Geometry: final body of the model. Coordinates: model frame, mm. A direction names the side the tool comes from. Give positions to 0.01 mm unless a question says otherwise; leave off trailing zeros. Write each loop counter-clockwise with the first axis right and the second up, starting at its lowest first coordinate (ties: lowest second). Pieces come first, ordered by that corner, then holes.
Q1. Cut plane A-A on z = 0. Return the cut outline in (x, y), plus the area to 3 significant figures.
Q2. Reachability of faces 1 (the face through (-7.5, 6, 2)), 2 (the face through (-2.81, 1, 0)), 3 (the face through (-6, 4, 10)) from +Z, -Z, +X, -X, +Y, -Y: full face, straight path, thin tool, end or side. Return the list, or none.
Q3. Cut plane D-D on x = 1.5. Return the cut outline in (y, z), plus the area to 3 significant figures.
Q4. Cut plane B-B on x = -8. Return the cut outline in (y, z), plus the area to 3 significant figures.
Q5. Line query: L1, parallel to Z at x = -9, y = 6; L2, parallel to Y at x = -8.15, z = 0; L3, parallel to Z at x = -6.75, y = 8.25. Output: solid intervals per line, ascending.
Q6. Cut plane C-C on y = 6. Return the cut outline in (x, z).
Q7. Pin query (flat end, axial travel): pin 1 (3.5 mm diameter, centred on y = 6, z = -4, fed in from +X); pin 2 (9 mm diameter, centred on x = 2, z = -2, fed in from +Y). Return the tip coordinate at first contact, or that it passes through.
Q8. Draft query along Y for faces 4 (the face through (-9, 10, 0)), 5 (the face through (-5, 4, -8)), 6 (the face through (-8.73, 6.97, -5.27)). Return one class per face: pulls with the +Y half, pulls with the -Y half, needs draft (parallel to the pull), parting line crosses it, or undercut.
```python
from build123d import *

# Parameters (mm, degrees)
SKETCH1_R           = 3.1
BOSS_EXTRUDE1_DEPTH = 2
BOSS_EXTRUDE2_DEPTH = 10
BOSS_EXTRUDE3_DEPTH = 2
BOSS_EXTRUDE4_DEPTH = 2
CUT_EXTRUDE1_DEPTH  = 5
BOSS_EXTRUDE5_START = -2
BOSS_EXTRUDE5_DEPTH = 2


with BuildPart() as part:
    # Sketch1 → Boss-Extrude1 (new body)
    with BuildSketch(Plane(origin=(0, 0, 0), x_dir=(1, 0, 0), z_dir=(0, 1, 0))):
        with BuildLine():
            ThreePointArc((0, -10), (10, 0), (0, 10))
            Line((0, 10), (-10, 10))
            Line((-10, 10), (-10, -10))
            Line((-10, -10), (0, -10))
        make_face()
        with Locations(Location((0, 0, 0), (0, 0, 270))):
            Circle(SKETCH1_R, mode=Mode.SUBTRACT)
    extrude(amount=BOSS_EXTRUDE1_DEPTH)

    # Sketch1<3> → Boss-Extrude2 (add)
    with BuildSketch(Plane(origin=(0, 0, 0), x_dir=(1, 0, 0), z_dir=(0, 1, 0))):
        with BuildLine():
            Line((-7.5, -6.614378278), (-7.5, 6.614378278))
            ThreePointArc((-7.5, 6.614378278), (-9.354143467, 3.535533906), (-10, 0))
            ThreePointArc((-10, 0), (-9.354143467, -3.535533906), (-7.5, -6.614378278))
        make_face()
        with BuildLine():
            Line((-7.5, 6.614378278), (-7.5, 10))
            Line((-7.5, 10), (-10, 10))
            Line((-10, 10), (-10, 0))
            ThreePointArc((-10, 0), (-9.354143467, 3.535533906), (-7.5, 6.614378278))
        make_face()
        with BuildLine():
            Line((-7.5, -10), (-7.5, -6.614378278))
            ThreePointArc((-7.5, -6.614378278), (-9.354143467, -3.535533906), (-10, 0))
            Line((-10, 0), (-10, -10))
            Line((-10, -10), (-7.5, -10))
        make_face()
    extrude(amount=BOSS_EXTRUDE2_DEPTH)

    # Sketch2 → Boss-Extrude3 (add)
    with BuildSketch(Plane.XY.offset(10)):
        Polygon((-7.5, 10), (0, 2), (-7.5, 2), align=None)
    extrude(amount=-BOSS_EXTRUDE3_DEPTH)

    # Sketch3 → Boss-Extrude4 (add)
    with BuildSketch(Plane(origin=(0, 0, -10), x_dir=(-1, 0, 0), z_dir=(0, 0, -1))):
        Polygon((0, 2), (7.5, 10), (7.5, 2), align=None)
    extrude(amount=-BOSS_EXTRUDE4_DEPTH)

    # Sketch4 → Cut-Extrude1 (cut)
    with BuildSketch(Plane(origin=(-7.5, 0, 0), x_dir=(0, 0, -1), z_dir=(1, 0, 0))):
        with BuildLine():
            ThreePointArc((-2.4, 6), (-4, 7.6), (-5.6, 6))
            Line((-5.6, 6), (-2.4, 6))
        make_face()
        with BuildLine():
            Line((-2.4, 6), (-5.6, 6))
            ThreePointArc((-5.6, 6), (-4, 4.4), (-2.4, 6))
        make_face()
        with BuildLine():
            ThreePointArc((1.6, 6), (0, 7.6), (-1.6, 6))
            Line((-1.6, 6), (0, 6))
            Line((0, 6), (1.6, 6))
        make_face()
        with BuildLine():
            Line((0, 6), (-1.6, 6))
            ThreePointArc((-1.6, 6), (0, 4.4), (1.6, 6))
            Line((1.6, 6), (0, 6))
        make_face()
        with BuildLine():
            ThreePointArc((5.6, 6), (4, 7.6), (2.4, 6))
            Line((2.4, 6), (5.6, 6))
        make_face()
        with BuildLine():
            Line((5.6, 6), (2.4, 6))
            ThreePointArc((2.4, 6), (4, 4.4), (5.6, 6))
        make_face()
    extrude(amount=-CUT_EXTRUDE1_DEPTH, mode=Mode.SUBTRACT)

    # Sketch5 → Boss-Extrude5 (add)
    with BuildSketch(Plane(origin=(0, 2, 0), x_dir=(1, 0, 0), z_dir=(0, 1, 0)).offset(BOSS_EXTRUDE5_START)):
        with BuildLine():
            Line((-2.81, -1.309160036), (-2.81, 0))
            Line((-2.81, 0), (-2.81, 1.309160036))
            ThreePointArc((-2.81, 1.309160036), (-3.1, 0), (-2.81, -1.309160036))
        make_face()
    extrude(amount=BOSS_EXTRUDE5_DEPTH)


solid = part.part
```
Data:
1. outline: (-10, 0) - (-2.81, 0) - (-2.81, 2) - (-7.5, 2) - (-7.5, 4.4) - (-10, 4.4) - close; (-10, 7.6) - (-7.5, 7.6) - (-7.5, 10) - (-10, 10) - close; (3.1, 0) - (10, 0) - (10, 2) - (3.1, 2) - close
1. area: 40.2 mm2
2. face 1: +X, +Y
2. face 2: +Y, -Y
2. face 3: +Z, +X, -X, +Y, -Y
3. outline: (0, -9.89) - (2, -9.89) - (2, -2.71) - (0, -2.71) - close; (0, 2.71) - (2, 2.71) - (2, 9.89) - (0, 9.89) - close
3. area: 28.7 mm2
4. outline: (0, -10) - (10, -10) - (10, 10) - (0, 10) - close; hole circle Ø3.2 at (6, -4); hole circle Ø3.2 at (6, 0); hole circle Ø3.2 at (6, 4)
4. area: 176 mm2
5. L1: z = -10 to -5.6, -2.4 to -1.6, 1.6 to 2.4, 5.6 to 10
5. L2: y = 0 to 4.4, 7.6 to 10
5. L3: z = -10 to -8, 8 to 10
6. outline: (-10, -10) - (-3.75, -10) - (-3.75, -8) - (-7.5, -8) - (-7.5, -5.6) - (-10, -5.6) - close; (-10, -2.4) - (-7.5, -2.4) - (-7.5, -1.6) - (-10, -1.6) - close; (-10, 1.6) - (-7.5, 1.6) - (-7.5, 2.4) - (-10, 2.4) - close; (-10, 5.6) - (-7.5, 5.6) - (-7.5, 8) - (-3.75, 8) - (-3.75, 10) - (-10, 10) - close
7. pin 1: stops at x = -7.5
7. pin 2: stops at y = 2
8. face 4: pulls with the +Y half
8. face 5: needs draft
8. face 6: undercut
